```python
from build123d import *

# Parameters (mm, degrees)
SCHIZZO1_W                   = 15
SCHIZZO1_H                   = 100
ESTRUSIONE_ESTRUSIONE1_DEPTH = 5
SCHIZZO2_W                   = 5
SCHIZZO2_H                   = 15
ESTRUSIONE_ESTRUSIONE2_DEPTH = 3
SCHIZZO4_R                   = 1.5
TAGLIO_ESTRUSIONE2_DEPTH     = 6
TAGLIO_ESTRUSIONE3_DEPTH     = 6
SCHIZZO6_R                   = 0.25
TAGLIO_ESTRUSIONE4_DEPTH     = 10


with BuildPart() as part:
    # Schizzo1 → Estrusione-Estrusione1 (new body)
    with BuildSketch(Plane(origin=(0, 0, 0), x_dir=(0, 0, -1), z_dir=(1, 0, 0))):
        Rectangle(SCHIZZO1_W, SCHIZZO1_H)
    extrude(amount=ESTRUSIONE_ESTRUSIONE1_DEPTH)

    # Schizzo2 → Estrusione-Estrusione2 (add)
    with BuildSketch(Plane(origin=(0, 0, -7.5), x_dir=(-1, 0, 0), z_dir=(0, 0, -1))):
        with Locations((-2.5, 22.5)):
            Rectangle(SCHIZZO2_W, SCHIZZO2_H)
        with Locations((-2.5, -22.5)):
            Rectangle(SCHIZZO2_W, SCHIZZO2_H)
    extrude(amount=ESTRUSIONE_ESTRUSIONE2_DEPTH)

    # Schizzo4 → Taglio-Estrusione2 (cut, through all)
    with BuildSketch(Plane(origin=(0, 0, 0), x_dir=(0, 0, -1), z_dir=(1, 0, 0))):
        with Locations((2.5, 30)):
            Circle(SCHIZZO4_R)
        with Locations((2.5, -30)):
            Circle(SCHIZZO4_R)
    extrude(amount=TAGLIO_ESTRUSIONE2_DEPTH, mode=Mode.SUBTRACT)

    # Schizzo5 → Taglio-Estrusione3 (cut, through all)
    with BuildSketch(Plane(origin=(5, 0, 0), x_dir=(0, 0, -1), z_dir=(1, 0, 0))):
        Polygon((-2.5, 1.25), (1.3, 1.25), (1.3, 2.75), (3.7, 2.75), (3.7, 1.25), (7.5, 1.25), (7.5, -1.25), (3.7, -1.25), (3.7, -2.75), (1.3, -2.75), (1.3, -1.25), (-2.5, -1.25), align=None)
        Polygon((-2.5, -38.75), (1.3, -38.75), (1.3, -37.25), (3.7, -37.25), (3.7, -38.75), (7.5, -38.75), (7.5, -41.25), (3.7, -41.25), (3.7, -42.75), (1.3, -42.75), (1.3, -41.25), (-2.5, -41.25), align=None)
        Polygon((7.5, 38.75), (7.5, 41.25), (3.7, 41.25), (3.7, 42.75), (1.3, 42.75), (1.3, 41.25), (-2.5, 41.25), (-2.5, 38.75), (1.3, 38.75), (1.3, 37.25), (3.7, 37.25), (3.7, 38.75), align=None)
    extrude(amount=-TAGLIO_ESTRUSIONE3_DEPTH, mode=Mode.SUBTRACT)

    # Schizzo6 → Taglio-Estrusione4 (cut)
    with BuildSketch(Plane(origin=(5, 0, 0), x_dir=(0, 0, -1), z_dir=(1, 0, 0))):
        with Locations((3.7, 42.75)):
            Circle(SCHIZZO6_R)
        with Locations((3.7, 37.25)):
            Circle(SCHIZZO6_R)
        with Locations((3.7, 2.75)):
            Circle(SCHIZZO6_R)
        with Locations((3.7, -2.75)):
            Circle(SCHIZZO6_R)
        with Locations((3.7, -37.25)):
            Circle(SCHIZZO6_R)
        with Locations((3.7, -42.75)):
            Circle(SCHIZZO6_R)
    extrude(amount=-TAGLIO_ESTRUSIONE4_DEPTH, mode=Mode.SUBTRACT)


solid = part.part
```
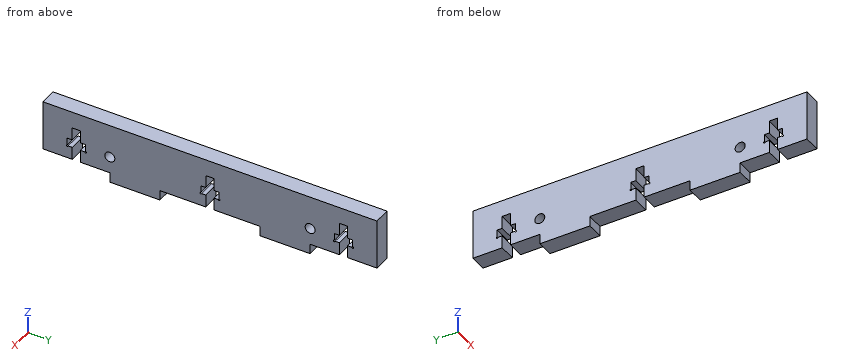
Geometry check sheet. Reference: the model listing, model coordinates, mm. Round coordinates to 2 decimals unless told otherwise and drop trailing zeros. Loops run counter-clockwise (first coordinate to the right, second up) from the corner with the lowest first, then second, coordinate; pieces in that order, holes last. Notation, with made-up numbers: (55, 2.5) - (83, 2.5) arc R26 cw to (83, 36.5) - close; hole circle Ø5 at (-18.75, 65). An arc over 180 degrees is marked (long way). Use a Markdown table: item, result.
Q1. Material ranges on line 1 (Y direction, x = 3.15, z = 2.25); line 2 (Y direction, x = 1.05, z = -2.5); line 3 (Y direction, x = 4.6, z = -10), recorded low to high.
Solutions:
| item | result |
|---|---|
| line 1 | y = -50 to -41.25, -38.75 to -1.25, 1.25 to 38.75, 41.25 to 50 |
| line 2 | y = -50 to -42.75, -37.25 to -31.5, -28.5 to -2.75, 2.75 to 28.5, 31.5 to 37.25, 42.75 to 50 |
| line 3 | y = -30 to -15, 15 to 30 |
Q2. Cross-section at A-A on z = -2.5. Record the cut outline in (x, y), plus the area to 4 significant figures.
Solutions:
| item | result |
|---|---|
| outline | (0, -50) - (5, -50) - (5, -42.75) - (0, -42.75) - close; (0, -37.25) - (5, -37.25) - (5, -31.5) - (0, -31.5) - close; (0, -28.5) - (5, -28.5) - (5, -2.75) - (0, -2.75) - close; (0, 2.75) - (5, 2.75) - (5, 28.5) - (0, 28.5) - close; (0, 31.5) - (5, 31.5) - (5, 37.25) - (0, 37.25) - close; (0, 42.75) - (5, 42.75) - (5, 50) - (0, 50) - close |
| area | 387.5 mm2 |
Q3. Go/stop test with a flat-tipped pin: P1, Ø2.5, axis at x = 2, y = 7, coming from the -Z side. Record where the tip stops, or that it passes through.
Solutions:
| item | result |
|---|---|
| P1 | stops at z = -7.5 |
Q4. Cross-section at B-B on x = 2.25. State how many separate pieces and enclosed holes the cut face has, plus the area to 3 significant figures.
Solutions:
| item | result |
|---|---|
| separate pieces | 1 |
| enclosed holes | 2 |
| area | 1,480 mm2 |
